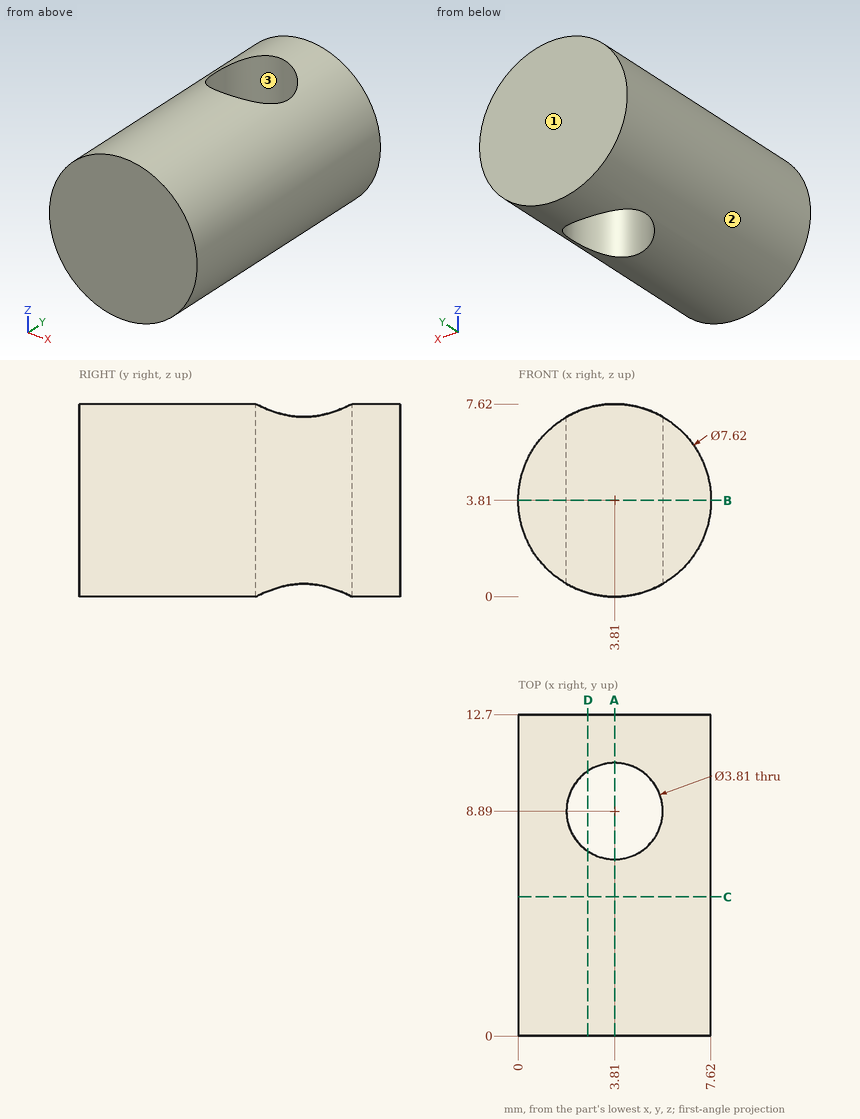
For this review, use the dimensioned drawing (mm, ordinates from the lowest corner) and the shaded views. Round coordinates to 2 decimals unless told otherwise and drop trailing zeros. Write each loop counter-clockwise with the first axis right and the second up, starting at its lowest first coordinate (ties: lowest second). Pieces come first, ordered by that corner, then holes. Notation, with made-up numbers: (55, -20.75) -> (84, -20.75) arc R29 ccw to (84, 12.25) -> close; hole circle Ø11 at (-37.5, -30). An arc over 180 degrees is marked (long way). One line per item, written item: value. Start each with the question number.
Q1. Insertion check: P1, Ø1.5, axis at y = 4, z = 5.5, coming from the -X side; P2, Ø3, axis at y = 3.5, z = 2.5, coming from the +X side. Each pin has a flat end and moves straight along its axis. Give the tip position at first contact, or say it passes through.
Q2. Add section B-B (z = 3.81). Give the boundary of the cut face in (x, y) (3 decimals), then the cut area to 3 significant figures.
Q3. The part is to be moulded in two halves that separate along X. For the marked faces 1, 2 and 3, say which applies: pulls with the +X half, pulls with the -X half, needs draft (parallel to the pull), parting line crosses it, or undercut.
Q4. To check wall thickness, follow probe 1 along Y at (x, z) = (3.81, 5) (3 decimals); probe 2 along Y at (x, z) = (5.5, 5.25); probe 3 along Z at (x, y) = (4.75, 7). State the ranges of each line that lie inside material, in increasing order.
Q5. Add section C-C (y = 5.5). Give the boundary of the cut face in (x, z).
Q6. Add section D-D (x = 2.75). Give the boundary of the cut face in (y, z).
Q7. Add section A-A (x = 3.81). Give the boundary of the cut face in (y, z) (3 decimals), then the cut area to 3 significant figures.
Response:
1. P1: stops at x = 0.12
1. P2: stops at x = 7.62
2. outline: (0, 0) -> (7.62, 0) -> (7.62, 12.7) -> (0, 12.7) -> close; hole circle Ø3.81 at (3.81, 8.89)
2. area: 85.4 mm^2
3. face 1: needs draft
3. face 2: parting line crosses it
3. face 3: undercut
4. probe 1: y = 0 to 6.985, 10.795 to 12.7
4. probe 2: y = 0 to 8.01, 9.77 to 12.7
4. probe 3: z = 0.12 to 7.5
5. outline: circle Ø7.62 at (3.81, 3.81)
6. outline: (0, 0.15) -> (7.31, 0.15) -> (7.31, 7.47) -> (0, 7.47) -> close; (10.47, 0.15) -> (12.7, 0.15) -> (12.7, 7.47) -> (10.47, 7.47) -> close
7. outline: (0, 0) -> (6.985, 0) -> (6.985, 7.62) -> (0, 7.62) -> close; (10.795, 0) -> (12.7, 0) -> (12.7, 7.62) -> (10.795, 7.62) -> close
7. area: 67.7 mm^2
